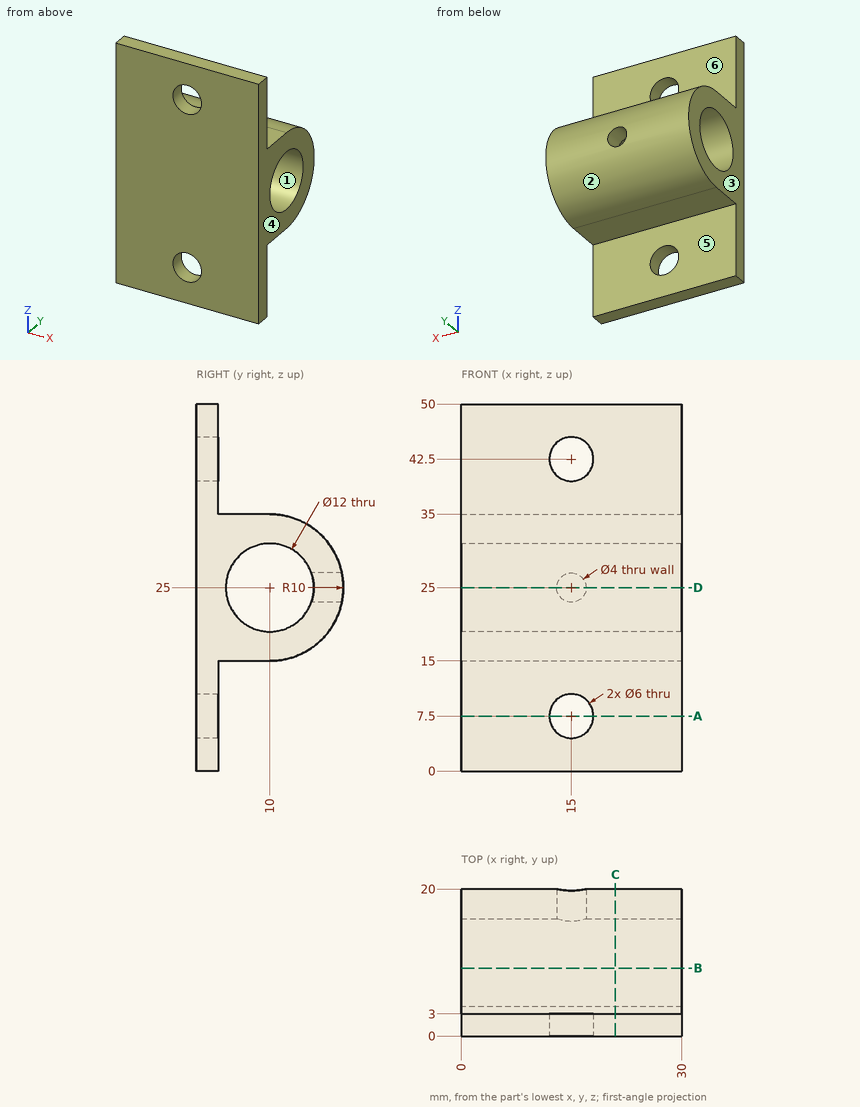
Can you work these out from the drawing? Everything is in mm from the part's minimum corner. A direction names the side the tool comes from. Give positions to 0.01 mm unless a question says otherwise; leave off trailing zeros. Order: outer loops, then holes, each group sorted by start corner. A loop starts at its lowest first (then second) coordinate and runs counter-clockwise, first axis right, second up. Notation, with made-up numbers: M -36,14 L -18,14 A26 cw -18,39 Z; hole C 65.25,77.25 d5. An arc over 180 degrees is marked long. One line per question, with ' | ' between items.
1. For the marked faces 4, 5 and 6, which set-ups out of +Z, -Z, +X, -X, +Y, -Y let a thin tool reach every point of the face, with its end or its side?
Results:
face 4: +Z, -Z, +X, +Y, -Y | face 5: -Z, +X, -X, +Y | face 6: +Z, +X, -X, +Y
2. I'm going to push flat-ended pins straight in: pin 1 (2 mm diameter, centred on x = 16, y = 7.5, fed in from +Z); pin 2 (7.5 mm diameter, centred on x = 21, z = 10, fed in from +Y); pin 3 (5 mm diameter, centred on x = 15, z = 42.5, fed in from -Y); pin 4 (6 mm diameter, centred on x = 6, y = 8.5, fed in from -Z). Where does each tip first touch, or does it pass through?
Results:
pin 1: z = 35 | pin 2: y = 3 | pin 3: through | pin 4: z = 15
3. We'd pull the mould along Y, two halves only. Please class the marked faces 1, 2 and 3: +Y half, -Y half, draft (parallel to the pull), parting line (faces both ways), or undercut.
Results:
face 1: undercut | face 2: +Y half | face 3: draft
4. I want a section at B-B (y = 9.25). List the corners of the cut face in (x, z) for me.
Results:
outline: M 0,15 L 30,15 L 30,19.05 L 0,19.05 Z; M 0,30.95 L 30,30.95 L 30,35 L 0,35 Z
5. I want a section at A-A (z = 7.5). List the corners of the cut face in (x, y) for me.
Results:
outline: M 0,0 L 12,0 L 12,3 L 0,3 Z; M 18,0 L 30,0 L 30,3 L 18,3 Z
6. I want a section at C-C (x = 21). List the corners of the cut face in (y, z) for me.
Results:
outline: M 0,0 L 3,0 L 3,15 L 10,15 A10 ccw 10,35 L 3,35 L 3,50 L 0,50 Z; hole C 10,25 d12
7. I want a section at D-D (z = 25). List the corners of the cut face in (x, y) for me, and give its area (3 significant figures).
Results:
outline: M 0,0 L 30,0 L 30,4 L 0,4 Z; M 0,16 L 13,16 L 13,20 L 0,20 Z; M 17,16 L 30,16 L 30,20 L 17,20 Z | area: 224 mm²
8. If I drill on line 1 (X direction, y = 1.05, z = 7.5); line 2 (Z direction, x = 15, y = 10); line 3 (Y direction, x = 4, z = 44), over which ranges is the centre line in solid material (lowest first)?
Results:
line 1: 0 to 12, 18 to 30 | line 2: 15 to 19, 31 to 35 | line 3: 0 to 3
